Source: CAD feature listing. Evaluate the final solid. Frame: model axes, mm. Face numbers are marked on the shaded views. Coordinates: 2 decimals unless noted, no trailing zeros. Write each loop counter-clockwise with the first axis right and the second up, starting at its lowest first coordinate (ties: lowest second). Pieces come first, ordered by that corner, then holes. Notation, with made-up numbers: (23, 2.25) -> (66, 2.25) arc R25 cw to (66, 14.25) -> close; hole circle Ø3 at (-17.5, -9.75). An arc over 180 degrees is marked (long way). Write item = value, one per line.
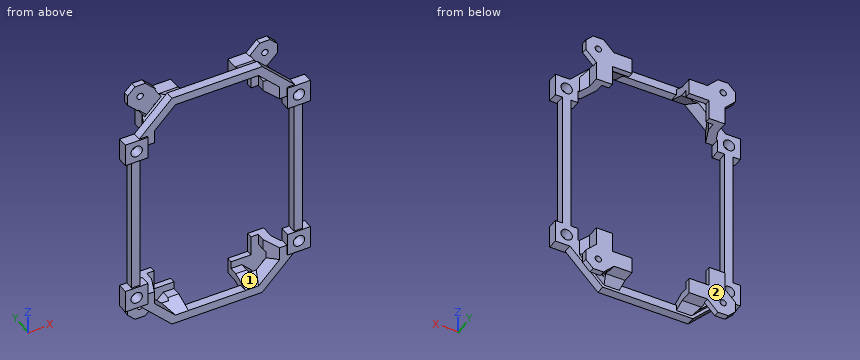
from build123d import *

# Parameters (mm, degrees)
BOSS_EXTRUDE1_DEPTH            = 6
BOSS_EXTRUDE2_DEPTH            = 1
BOSS_EXTRUDE3_DEPTH            = 12.05
SKETCH4_R                      = 2.25
BOSS_EXTRUDE4_DEPTH            = 4
CUT_EXTRUDE1_REACH             = 87.707
SKETCH5_W                      = 16.364675298
SKETCH5_H                      = 8
CUT_EXTRUDE1_DIRECTION_2_DEPTH = 86.707273439
CUT_EXTRUDE2_DEPTH             = 9.171573
CUT_EXTRUDE3_REACH             = 114.79
SKETCH8_W                      = 3.39411255
SKETCH8_H                      = 10.05
CUT_EXTRUDE3_DIRECTION_2_REACH = 114.79
BOSS_EXTRUDE5_DEPTH            = 13.628427
CUT_EXTRUDE4_DEPTH             = 113.7898768
SKETCH12_R                     = 4.0132
CUT_EXTRUDE5_DEPTH             = 113.888407941


with BuildPart() as part:
    # Sketch1 → Boss-Extrude1 (new body)
    with BuildSketch(Plane(origin=(0, 0, 0), x_dir=(1, 0, 0), z_dir=(0, 1, 0))):
        Polygon((-54.15, 0), (-60.15, 0), (-60.15, -49.15), (-65.15, -49.15), (-65.15, -65.15), (-54.806854249, -65.15), (-31.756854249, -88.2), (0, -88.2), (0, -82.2), (-20.1, -82.2), (-20.1, -77.4), (-31.243145751, -77.4), (-39.3, -69.343145751), (-39.3, -58.2), (-49.15, -58.2), (-49.15, -49.15), (-54.15, -49.15), align=None)
    extrude(amount=BOSS_EXTRUDE1_DEPTH)

    # Sketch2 → Boss-Extrude2 (add)
    with BuildSketch(Plane.XZ):
        Polygon((-49.15, 58.2), (-49.15, 49.15), (-65.15, 49.15), (-65.15, 65.15), (-49.15, 65.15), align=None)
    extrude(amount=BOSS_EXTRUDE2_DEPTH)

    # Sketch3 → Boss-Extrude3 (add)
    with BuildSketch(Plane(origin=(0, 6, 0), x_dir=(1, 0, 0), z_dir=(0, 1, 0))):
        Polygon((-39.3, -58.2), (-45.3, -58.2), (-45.3, -71.828427125), (-33.728427125, -83.4), (-20.1, -83.4), (-20.1, -77.4), (-31.243145751, -77.4), (-39.3, -69.343145751), align=None)
    extrude(amount=BOSS_EXTRUDE3_DEPTH)

    # Sketch4 → Boss-Extrude4 (add)
    with BuildSketch(Plane(origin=(0, 18.05, 0), x_dir=(1, 0, 0), z_dir=(0, 1, 0))):
        Polygon((-45.3, -58.2), (-34.1, -58.2), (-34.1, -72.2), (-20.1, -72.2), (-20.1, -83.4), (-32.925631329, -83.4), (-40.309262274, -90.783630945), (-47.557999616, -90.783630945), (-52.683630945, -85.657999616), (-52.683630945, -78.409262274), (-45.3, -71.025631329), align=None)
        with Locations(Location((-43.933630945, -82.033630945, 0), (0, 0, 270))):
            Circle(SKETCH4_R, mode=Mode.SUBTRACT)
    extrude(amount=BOSS_EXTRUDE4_DEPTH)

    # Sketch5 → Cut-Extrude1 (cut, up to next)
    with BuildSketch(Plane(origin=(-58.564213562, 0, 58.564213562), x_dir=(0.7071067811865475, 0, 0.7071067811865477), z_dir=(-0.7071067811865477, 0, 0.7071067811865475)), mode=Mode.PRIVATE) as cut_extrude1_sk1:
        with Locations((26.940768363, 14.05)):
            Rectangle(SKETCH5_W, SKETCH5_H)
    cut_extrude1_tool1 = extrude(cut_extrude1_sk1.sketch, amount=-CUT_EXTRUDE1_REACH, mode=Mode.PRIVATE) & part.part
    add(cut_extrude1_tool1.solids().sort_by_distance((-39.514214, 14.05, 77.614214))[0], mode=Mode.SUBTRACT)

    # Sketch5 → Cut-Extrude1 direction 2 (cut)
    with BuildSketch(Plane(origin=(-58.564213562, 0, 58.564213562), x_dir=(0.7071067811865475, 0, 0.7071067811865477), z_dir=(-0.7071067811865477, 0, 0.7071067811865475))):
        with Locations((26.940768363, 14.05)):
            Rectangle(SKETCH5_W, SKETCH5_H)
    extrude(amount=CUT_EXTRUDE1_DIRECTION_2_DEPTH, mode=Mode.SUBTRACT)

    # Sketch6 → Cut-Extrude2 (cut)
    with BuildSketch(Plane(origin=(-20.1, 0, 0), x_dir=(0, 0, -1), z_dir=(1, 0, 0))):
        Polygon((-82.2, 0), (-77.4, 12.05), (-77.4, 0), align=None)
    cut_extrude2 = extrude(amount=-CUT_EXTRUDE2_DEPTH, mode=Mode.SUBTRACT)

    # Mirror1: Cut-Extrude2 across plane
    add(cut_extrude2.mirror(Plane(origin=(19.05, 0, 19.05), x_dir=(-0.7071067811865477, 0, 0.7071067811865474), z_dir=(0.7071067811865476, 0, 0.7071067811865476))), mode=Mode.SUBTRACT)

    # Cut-Extrude3: up to this plane
    cut_extrude3_end = Plane(origin=(-44.1, 0, 67.371572875), z_dir=(0.9290074363039443, -0.3700610534654694, 0))
    # Sketch8 → Cut-Extrude3 (cut, up to the surface)
    with BuildSketch(Plane(origin=(19.05, 0, 19.05), x_dir=(0.7071067811865476, 0, -0.7071067811865476), z_dir=(0.7071067811865476, 0, 0.7071067811865476)), mode=Mode.PRIVATE) as cut_extrude3_sk1:
        with Locations((-77.125248815, 5.025)):
            Rectangle(SKETCH8_W, SKETCH8_H)
    cut_extrude3_tool1 = split(extrude(cut_extrude3_sk1.sketch, amount=-CUT_EXTRUDE3_REACH, mode=Mode.PRIVATE), bisect_by=cut_extrude3_end, keep=Keep.BOTH, mode=Mode.PRIVATE)
    add(cut_extrude3_tool1.solids().sort_by_distance((-35.485786, 5.025, 73.585786))[0], mode=Mode.SUBTRACT)

    # Cut-Extrude3 direction 2: up to this plane
    cut_extrude3_direction_2_end = Plane(origin=(-29.271572875, 0, 82.2), z_dir=(0, 0.3700610534654694, 0.9290074363039443))
    # Sketch8 → Cut-Extrude3 direction 2 (cut, up to the surface)
    with BuildSketch(Plane(origin=(19.05, 0, 19.05), x_dir=(0.7071067811865476, 0, -0.7071067811865476), z_dir=(0.7071067811865476, 0, 0.7071067811865476)), mode=Mode.PRIVATE) as cut_extrude3_direction_2_sk1:
        with Locations((-77.125248815, 5.025)):
            Rectangle(SKETCH8_W, SKETCH8_H)
    cut_extrude3_direction_2_tool1 = split(extrude(cut_extrude3_direction_2_sk1.sketch, amount=CUT_EXTRUDE3_DIRECTION_2_REACH, mode=Mode.PRIVATE), bisect_by=cut_extrude3_direction_2_end, keep=Keep.BOTH, mode=Mode.PRIVATE)
    add(cut_extrude3_direction_2_tool1.solids().sort_by_distance((-35.485786, 5.025, 73.585786))[0], mode=Mode.SUBTRACT)

    # Sketch10 → Boss-Extrude5 (add)
    with BuildSketch(Plane(origin=(-20.1, 0, 0), x_dir=(0, 0, -1), z_dir=(1, 0, 0))):
        Polygon((-83.4, 13.20104083), (-86.268464397, 6), (-83.4, 6), align=None)
    boss_extrude5 = extrude(amount=-BOSS_EXTRUDE5_DEPTH)

    # Sketch11 → Cut-Extrude4 (cut, through all)
    with BuildSketch(Plane(origin=(19.05, 0, 19.05), x_dir=(0.7071067811865476, 0, -0.7071067811865476), z_dir=(0.7071067811865476, 0, 0.7071067811865476))):
        Polygon((-82.82230509, 13.20104083), (-84.850615716, 6), (-82.82230509, 6), align=None)
    cut_extrude4 = extrude(amount=CUT_EXTRUDE4_DEPTH, mode=Mode.SUBTRACT)

    # Mirror2: Boss-Extrude5, Cut-Extrude4 across plane
    add(boss_extrude5.mirror(Plane(origin=(19.05, 0, 19.05), x_dir=(-0.7071067811865477, 0, 0.7071067811865474), z_dir=(0.7071067811865476, 0, 0.7071067811865476))))
    add(cut_extrude4.mirror(Plane(origin=(19.05, 0, 19.05), x_dir=(-0.7071067811865477, 0, 0.7071067811865474), z_dir=(0.7071067811865476, 0, 0.7071067811865476))), mode=Mode.SUBTRACT)

    # Sketch12 → Cut-Extrude5 (cut, through all)
    with BuildSketch(Plane(origin=(0, 6, 0), x_dir=(1, 0, 0), z_dir=(0, 1, 0))):
        with Locations(Location((-57.15, -57.15, 0), (0, 0, 270))):
            Circle(SKETCH12_R)
    extrude(amount=-CUT_EXTRUDE5_DEPTH, mode=Mode.SUBTRACT)

    # Mirror3: part across plane


with BuildPart() as part_1:
    add(part.part)
    add(part.part.mirror(Plane(origin=(-54.15, 6, 0), x_dir=(1, 0, 0), z_dir=(0, 0, 1))))

    # Mirror4: part across plane


with BuildPart() as part_2:
    add(part_1.part)
    add(part_1.part.mirror(Plane(origin=(0, 6, -88.2), x_dir=(0, 0, 1), z_dir=(-1, 0, 0))))


solid = part_2.part
1) Cut plane D-D, the plane x = 2.5. Output: boundary loops of the cut face in (y, z).
Answer block:
outline = (0, -88.2) -> (6, -88.2) -> (6, -82.2) -> (0, -82.2) -> close; (0, 82.2) -> (6, 82.2) -> (6, 88.2) -> (0, 88.2) -> close
2) First-contact query: pin 1 Ø3 at (x, y) = (23, 14) entering from +Z; pin 2 Ø10.5 at (x, z) = (57.15, -57.15) entering from +Y; pin 3 Ø1.2 at (y, z) = (20.5, -66) entering from +X; pin 4 Ø6.5 at (x, z) = (57.15, 57.15) entering from -Y. Flat tips, straight axial feed; report the tip coordinate or a pass-through.
Answer block:
pin_1 = 83.68
pin_2 = 6
pin_3 = 45.3
pin_4 = through
3) Cut plane B-B, the plane x = -57.15. Output: boundary loops of the cut face in (y, z).
Answer block:
outline = (-1, -65.15) -> (6, -65.15) -> (6, -61.16) -> (-1, -61.16) -> close; (-1, -53.14) -> (6, -53.14) -> (6, 53.14) -> (-1, 53.14) -> (-1, 49.15) -> (0, 49.15) -> (0, -49.15) -> (-1, -49.15) -> close; (-1, 61.16) -> (6, 61.16) -> (6, 65.15) -> (-1, 65.15) -> close
4) Cut plane C-C, the plane y = 15.75. Give the number of separate pieces and of enclosed holes in the cut face, and give its area (3 significant figures).
Answer block:
separate_pieces = 8
enclosed_holes = 0
area = 510 mm2
5) Material intervals for probe 1 along Z at (x, y) = (57.15, 1); probe 2 along X at (y, z) = (1, -57.15); probe 3 along Z at (x, y) = (-26, 18.5), sorted ascending. Write a range as [from, to].
Answer block:
probe_1 = [-65.15, -61.16], [-53.14, 53.14], [61.16, 65.15]
probe_2 = [-65.15, -61.16], [-53.14, -49.15], [49.15, 53.14], [61.16, 65.15]
probe_3 = [-83.4, -72.2], [72.2, 83.4]
6) Pull-direction query (X, two-part tool) for the marked faces 1 and 2; classes: +X half, -X half, draft (parallel to the pull), parting line (faces both ways), or undercut.
Answer block:
face_1 = undercut
face_2 = draft
7) Cut plane A-A, the plane z = 41. Output: boundary loops of the cut face in (x, y), and give its area (3 significant figures).
Answer block:
outline = (-60.15, 0) -> (-54.15, 0) -> (-54.15, 6) -> (-60.15, 6) -> close; (54.15, 0) -> (60.15, 0) -> (60.15, 6) -> (54.15, 6) -> close
area = 72.0 mm2
